from build123d import *

# Parameters (mm, degrees)
EXTRUDE_1_DEPTH     = 800
SKETCH_2_R          = 5
CUT_EXTRUDE_3_DEPTH = 10


with BuildPart() as part:
    # Эскиз1 → Вытянуть-Тонкостенный1 (new body)
    with BuildSketch(Plane.XY):
        Polygon((0, 25), (0, 0), (25, 0), (25, -3), (-3, -3), (-3, 25), align=None)
    extrude(amount=EXTRUDE_1_DEPTH)

    # Эскиз2 → Вырез-Вытянуть3 (cut)
    with BuildSketch(Plane.YZ.offset(-3)):
        with Locations((10, 780)):
            Circle(SKETCH_2_R)
    extrude(amount=CUT_EXTRUDE_3_DEPTH, mode=Mode.SUBTRACT)


solid = part.part
Could you check a few things on this model? Use its own coordinates, in mm. A direction names the side the tool comes from. Round coordinates to 2 decimals unless told otherwise and drop trailing zeros. Order: outer loops, then holes, each group sorted by start corner. A loop starts at its lowest first (then second) coordinate and runs counter-clockwise, first axis right, second up.
(1) Imagine slicing it at B-B (z = 564.5). Write out the boundary of the cut face in (x, y), plus the area to 3 significant figures.
Response values:
outline: (-3, -3) - (25, -3) - (25, 0) - (0, 0) - (0, 25) - (-3, 25) - close
area: 159 mm2
(2) I'm going to push flat-ended pins straight in: pin 1 (7.5 mm diameter, centred on x = 17.5, z = 478.5, fed in from +Y); pin 2 (2 mm diameter, centred on y = 15.5, z = 193, fed in from +X). Where does each tip first touch, or does it pass through?
Response values:
pin 1: stops at y = 0
pin 2: stops at x = 0
(3) Imagine slicing it at C-C (x = 9). Write out the boundary of the cut face in (y, z), plus the area to 3 significant figures.
Response values:
outline: (-3, 0) - (0, 0) - (0, 800) - (-3, 800) - close
area: 2,400 mm2
(4) Which directions (+Z, -Z, +X, -X, +Y, -Y) give clear straight access to the entire face, cutting with the end or side of a thin tool? Please do faces 1 (the flat face through (11, -3, 394)), 2 (the flat face through (12, 0, 394)).
Response values:
face 1: +Z, -Z, +X, -X, -Y
face 2: +Z, -Z, +X, +Y
(5) Please list where these lines run through material, in increasing order: line 1 along Y through (x, z) = (-1.05, 780); line 2 along Z through (x, y) = (-2.35, 10); line 3 along X through (y, z) = (23.25, 55).
Response values:
line 1: y = -3 to 5, 15 to 25
line 2: z = 0 to 775, 785 to 800
line 3: x = -3 to 0
(6) Imagine slicing it at A-A (y = 10). Write out the boundary of the cut face in (x, z).
Response values:
outline: (-3, 0) - (0, 0) - (0, 775) - (-3, 775) - close; (-3, 785) - (0, 785) - (0, 800) - (-3, 800) - close
